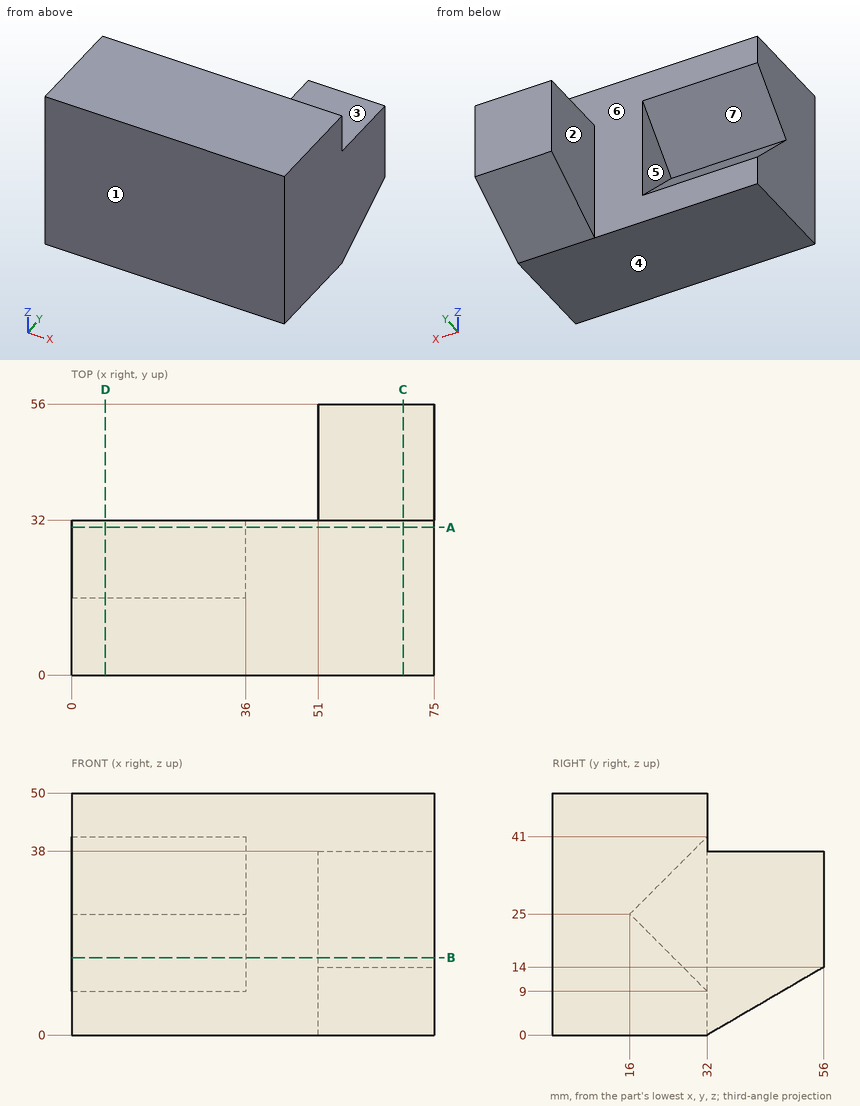
Drawing for the job (mm, zero at the part's lowest x, y, z). A direction names the side the tool comes from. Give positions to 0.01 mm unless a question says otherwise; leave off trailing zeros. Write each loop counter-clockwise with the first axis right and the second up, starting at its lowest first coordinate (ties: lowest second). Pieces come first, ordered by that corner, then holes. Notation, with made-up numbers: (37, 80.5) -> (94, 80.5) arc R29 cw to (94, 115.5) -> close; hole circle Ø9 at (0, 16.25). An arc over 180 degrees is marked (long way). Put each result on its own line as item: value. Start each with the question number.
Item 1: Cut at A-A (y = 30.5). List the corners of the cut face in (x, z).
Item 2: Cut at D-D (x = 7). List the corners of the cut face in (y, z).
Item 3: Which spindle directions (+Z, -Z, +X, -X, +Y, -Y) get a long thin tool onto all of the face, cutting with end or side? Do the marked faces 1, 2 and 3. Say none if no direction does.
Item 4: Wall check: L1, parallel to X at y = 38, z = 37; L2, parallel to X at y = 31.5, z = 24; L3, parallel to Y at x = 38, z = 43. Give the ranges that are in metal, low to high. Write a range as [from, to].
Item 5: Cut at C-C (x = 68.5). List the corners of the cut face in (y, z), then the cut area to 3 significant figures.
Item 6: Pin check, flat tips, straight feed: pin 1 Ø5 at (y, z) = (37.5, 19) entering from -X; pin 2 Ø25 at (x, z) = (28.5, 18) entering from +Y. Stop position of each tip, or through.
Item 7: Pull direction Z, two halves, no side cores. Call the marked faces 4, 5, 6 and 7: pulls with the +Z half, pulls with the -Z half, needs draft (parallel to the pull), parting line crosses it, or undercut.
Item 8: Cut at B-B (z = 16). List the corners of the cut face in (x, y).
Answer list:
1. outline: (0, 0) -> (75, 0) -> (75, 50) -> (0, 50) -> (0, 39.5) -> (36, 39.5) -> (36, 10.5) -> (0, 10.5) -> close
2. outline: (0, 0) -> (32, 0) -> (32, 9) -> (16, 25) -> (32, 41) -> (32, 50) -> (0, 50) -> close
3. face 1: +Z, -Z, +X, -X, -Y
3. face 2: +Z, -Z, -X, +Y
3. face 3: +Z, +X, -X, +Y
4. L1: x = [51, 75]
4. L2: x = [36, 75]
4. L3: y = [0, 32]
5. outline: (0, 0) -> (32, 0) -> (56, 14) -> (56, 38) -> (32, 38) -> (32, 50) -> (0, 50) -> close
5. area: 2,340 mm2
6. pin 1: stops at x = 51
6. pin 2: stops at y = 32
7. face 4: pulls with the -Z half
7. face 5: undercut
7. face 6: needs draft
7. face 7: undercut
8. outline: (0, 0) -> (75, 0) -> (75, 56) -> (51, 56) -> (51, 32) -> (36, 32) -> (36, 25) -> (0, 25) -> close
